Geometry: final body of the model. Coordinates: model frame, mm. A direction names the side the tool comes from. Coordinates: 2 decimals unless noted, no trailing zeros. Loops run counter-clockwise (first coordinate to the right, second up) from the corner with the lowest first, then second, coordinate; pieces in that order, holes last. Notation, with made-up numbers: (70.25, -14.75) - (129.25, -14.75) arc R22 ccw to (129.25, -1.75) - close; hole circle Ø5 at (51, 68). An arc over 180 degrees is marked (long way). Put each result on its own line as item: value. Start each with the question number.
1) Section C-C on y = -9.25. Output: boundary loops of the cut face in (x, z).
2) Section B-B on y = -2.5. Output: boundary loops of the cut face in (x, z).
3) Draft query along Z for faces 1 (the cylindrical face through (3, -2, 0)), 2 (the flat face through (1.299, -1, 0)), 3 (the flat face through (-1.3, -3.315, 1.3)). Return one class per face: +Z half, -Z half, draft (parallel to the pull), parting line (faces both ways), or undercut.
4) Contact query for flat-ended pins moving along their axis: pin 1 Ø1 at (y, z) = (-7, 0.5) entering from +X; pin 2 Ø3 at (x, z) = (0.5, 0.5) entering from +Y; pin 3 Ø2 at (x, y) = (-2, -9.5) entering from +Z; pin 4 Ø1 at (x, y) = (0.5, -5.5) entering from -Z. Output: stop coordinate, or through.
5) Section A-A on z = 0. Output: boundary loops of the cut face in (x, y).
6) Material intervals for line 1 along Y through (x, z) = (1.7, 0.8); line 2 along Y through (x, z) = (-0.55, 0.3); line 3 along Z through (x, y) = (0.45, -1.25), sorted ascending. Write a range as from..to.
7) Reachability of faces 4 (the flat face through (0, -2.315, 0)), 5 (the flat face through (-1.1, -0.315, 1.1)), 6 (the cylindrical face through (1.5, -8.24, 0.07)) from +Z, -Z, +X, -X, +Y, -Y: full face, straight path, thin tool, end or side. Return the list, or none.
Autodesk Inventor part; units mm, degrees
ref_plane "YZ Plane" through (0, 0, 0) normal (1, 0, 0) x (0, 1, 0)
ref_plane "XZ Plane" through (0, 0, 0) normal (0, 1, 0) x (-1, 0, 0)
ref_plane "XY Plane" through (0, 0, 0) normal (0, 0, 1) x (1, 0, 0)
sketch "スケッチ1" plane through (0, 0, 0) normal (0, 0, 1) x (1, 0, 0)
  line L0 (-3, -0.3147) -> (0, -0.3147)
  line L1 (0, -0.3147) -> (0, -3.3147)
  line L2 (0, -3.3147) -> (-3, -3.3147)
  line L3 (-3, -3.3147) -> (-3, -0.3147)
  line L4 (-1.5, -3.3147) -> (0, -3.3147)
  line L5 (0, -3.3147) -> (0, -13.3147)
  line L6 (0, -13.3147) -> (-1.5, -13.3147)
  line L7 (-1.5, -13.3147) -> (-1.5, -3.3147)
  point P0 (0, 0)
  dimension "d0" = 1.5
  dimension "d1" = 0
  dimension "d2" = 10
  dimension "d3" = 0
  dimension "d4" = 3
revolve "回転1" add sketch "スケッチ1" angle 360 about axis through (0, -3.3147, 0) along (0, -1, 0)
thread "ねじ1"
sketch "スケッチ2" plane through (0, -0.3147, 0) normal (0, 1, 0) x (1, 0, 0)
  circle A0 centre (0, 0) radius 3
  line L0 (0, 1.5) -> (1.299, 0.75)
  line L1 (1.299, 0.75) -> (1.299, -0.75)
  line L2 (1.299, -0.75) -> (0, -1.5)
  line L3 (0, -1.5) -> (-1.299, -0.75)
  line L4 (-1.299, -0.75) -> (-1.299, 0.75)
  line L5 (-1.299, 0.75) -> (0, 1.5)
  dimension "d8" = 1.5
extrude "押し出し1" cut sketch "スケッチ2" against normal blind 2 contours L0 L1 L2 L3 L4 L5
fillet "フィレット1" radius 0.5 1 edges at (3, -0.3147, 0)
properties part number "M3_10" material "アルミニウム 6061"
Answer block:
1. outline: circle Ø3 at (0, 0)
2. outline: circle Ø6 at (0, 0)
3. face 1: parting line
3. face 2: undercut
3. face 3: draft
4. pin 1: stops at x = 1.5
4. pin 2: stops at y = -0.31
4. pin 3: stops at z = 1.12
4. pin 4: stops at z = -1.5
5. outline: (-3, -3.31) - (-1.5, -3.31) - (-1.5, -13.31) - (1.5, -13.31) - (1.5, -3.31) - (3, -3.31) - (3, -0.81) arc R0.5 ccw to (2.5, -0.31) - (1.3, -0.31) - (1.3, -2.31) - (-1.3, -2.31) - (-1.3, -0.31) - (-2.5, -0.31) arc R0.5 ccw to (-3, -0.81) - close
6. line 1: y = -3.31..-0.31
6. line 2: y = -13.31..-2.31
6. line 3: z = -2.97..-1.24, 1.24..2.97
7. face 4: +Y
7. face 5: +Z, -Z, +X, -X, +Y
7. face 6: -Y
